from build123d import *

# Parameters (mm, degrees)
CROQUIS1_W                              = 42
CROQUIS1_H                              = 12
SALIENTE_EXTRUIR1_DEPTH                 = 10
CORTAR_EXTRUIR1_DEPTH                   = 27.172504657
DI_METRO_DE_TALADRO_5_0_5_1_D           = 5
DI_METRO_DE_TALADRO_5_0_5_1_CSINK_D     = 10.999999995
DI_METRO_DE_TALADRO_5_0_5_1_CSINK_ANGLE = 90
DI_METRO_DE_TALADRO_3_5_3_5_1_D         = 3.5
REDONDEO1_R                             = 0.5


with BuildPart() as part:
    # Croquis1 → Saliente-Extruir1 (new body)
    with BuildSketch(Plane.XZ):
        with Locations((0, 6)):
            Rectangle(CROQUIS1_W, CROQUIS1_H)
    extrude(amount=-SALIENTE_EXTRUIR1_DEPTH)

    # Croquis2 → Cortar-Extruir1 (cut, through all)
    with BuildSketch(Plane(origin=(0, 0, 0), x_dir=(-1, 0, 0), z_dir=(0, 0, -1))):
        with BuildLine():
            Line((-6.883596498, 0), (6.883596498, 0))
            ThreePointArc((6.883596498, 0), (0, 2.952779272), (-6.883596498, 0))
        make_face()
    extrude(amount=-CORTAR_EXTRUIR1_DEPTH, mode=Mode.SUBTRACT)

    # Diámetro de taladro Ø5.0 (5)1 (through all)
    with Locations(Plane(origin=(0, 0, 0), x_dir=(-1, 0, 0), z_dir=(0, -1, 0))):
        with Locations((10, -6), (-10, -6)):
            CounterSinkHole(DI_METRO_DE_TALADRO_5_0_5_1_D / 2, DI_METRO_DE_TALADRO_5_0_5_1_CSINK_D / 2, counter_sink_angle=DI_METRO_DE_TALADRO_5_0_5_1_CSINK_ANGLE)

    # Diámetro de taladro Ø3.5 (3.5)1 (through all)
    with Locations(Plane(origin=(0, 0, 0), x_dir=(-1, 0, 0), z_dir=(0, 0, -1))):
        with Locations((15.5, 4.5), (-15.5, 4.5)):
            Hole(DI_METRO_DE_TALADRO_3_5_3_5_1_D / 2)

    # Redondeo1
    redondeo1_edges = [part.edges().sort_by_distance(p)[0] for p in [
        (21, 10, 6),
        (13.941798249, 0, 0),
        (-13.941798249, 0, 12),
        (0, 10, 12),
        (0, 2.952779272, 12),
        (0, 2.952779272, 0),
        (-21, 10, 6),
        (13.941798249, 0, 12),
        (21, 0, 6),
        (-13.941798249, 0, 0),
        (-21, 0, 6),
        (-21, 5, 12),
        (21, 5, 12),
        (21, 5, 0),
        (-21, 5, 0),
        (0, 10, 0),
    ]]
    fillet(redondeo1_edges, radius=REDONDEO1_R)


solid = part.part
Here's how the part is built. I have some questions about the finished solid (model axes, mm). Coordinates: 2 decimals unless noted, no trailing zeros. Order: outer loops, then holes, each group sorted by start corner. A loop starts at its lowest first (then second) coordinate and runs counter-clockwise, first axis right, second up. Notation, with made-up numbers: (22.25, 32) -> (41.25, 32) arc R22 ccw to (41.25, 54) -> close; hole circle Ø6 at (58, 2). An arc over 180 degrees is marked (long way). Answer in a Markdown table with one row per item.
(1) I want a section at A-A on y = 4.5. List the corners of the cut face in (x, z) for me, then the cut area to 3 significant figures.
Answer key:
| item | result |
|---|---|
| outline | (-21, 0.5) arc R0.5 ccw to (-20.5, 0) -> (-17.25, 0) -> (-17.25, 12) -> (-20.5, 12) arc R0.5 ccw to (-21, 11.5) -> close; (-13.75, 0) -> (13.75, 0) -> (13.75, 12) -> (-13.75, 12) -> close; (17.25, 0) -> (20.5, 0) arc R0.5 ccw to (21, 0.5) -> (21, 11.5) arc R0.5 ccw to (20.5, 12) -> (17.25, 12) -> close; hole circle Ø5 at (-10, 6); hole circle Ø5 at (10, 6) |
| area | 381 mm^2 |
(2) I want a section at C-C on y = 2. Count the separate pieces of the cut face and the enclosed holes in it, then the cut area to 3 significant figures.
Answer key:
| item | result |
|---|---|
| separate pieces | 2 |
| enclosed holes | 2 |
| area | 327 mm^2 |
(3) Please list where these lines run through material, in increasing order: probe 1 along Y at (x, z) = (15.5, 7.5); probe 2 along X at (y, z) = (5, 2); probe 3 along X at (y, z) = (1.5, 4).
Answer key:
| item | result |
|---|---|
| probe 1 | 0 to 2.75, 6.25 to 10 |
| probe 2 | -21 to -17.18, -13.82 to 13.82, 17.18 to 21 |
| probe 3 | -21 to -13.46, -6.54 to -5.05, 5.05 to 6.54, 13.46 to 21 |
(4) Thinking about a two-plate mould opening in Z: for faces 1 (the face through (0, 5, 0)), 2 (the face through (0, 5, 12)), 3 (the face through (-11.84, 6.55, 4.31)), 4 (the face through (17, 0, 6)), which applies, +Z half, -Z half, draft (parallel to the pull), parting line (faces both ways), or undercut?
Answer key:
| item | result |
|---|---|
| face 1 | -Z half |
| face 2 | +Z half |
| face 3 | undercut |
| face 4 | draft |
(5) I want a section at B-B on z = 6. List the corners of the cut face in (x, y) for me, then the cut area to 3 significant figures.
Answer key:
| item | result |
|---|---|
| outline | (-21, 0.5) arc R0.5 ccw to (-20.5, 0) -> (-15.5, 0) -> (-12.5, 3) -> (-12.5, 10) -> (-20.5, 10) arc R0.5 ccw to (-21, 9.5) -> close; (-7.5, 3) -> (-5.62, 1.12) arc R9.5 cw to (5.62, 1.12) -> (7.5, 3) -> (7.5, 10) -> (-7.5, 10) -> close; (12.5, 3) -> (15.5, 0) -> (20.5, 0) arc R0.5 ccw to (21, 0.5) -> (21, 9.5) arc R0.5 ccw to (20.5, 10) -> (12.5, 10) -> close; hole circle Ø3.5 at (-15.5, 4.5); hole circle Ø3.5 at (15.5, 4.5) |
| area | 257 mm^2 |
(6) Will this pin go through, and if not, where does the flat tip stop? pin 1 Ø6.5 at (x, z) = (10, 6) entering from -Y.
Answer key:
| item | result |
|---|---|
| pin 1 | y = 2.25 |
